Autodesk Inventor part; units mm, degrees
ref_plane "YZ Plane" through (0, 0, 0) normal (1, 0, 0) x (0, 1, 0)
ref_plane "XZ Plane" through (0, 0, 0) normal (0, 1, 0) x (-1, 0, 0)
ref_plane "XY Plane" through (0, 0, 0) normal (0, 0, 1) x (1, 0, 0)
sketch "Sketch1" plane through (0, 0, 0) normal (0, 0, 1) x (1, 0, 0)
  line L0 (210, -0.4421) -> (210, 134.5579)
  line L1 (210, 134.5579) -> (70, 134.5579)
  line L2 (0, 60) -> (0, 0)
  line L3 (70, 60) -> (0, 60)
  line L4 (0, 60) -> (0, 0)
  line L5 (70, 60) -> (70, 134.5579)
  line L6 (0, 0) -> (24.7692, 0)
  line L7 (70, -0.4421) -> (70, 134.5579) construction
  arc A0 (184.7692, 18.0579) -> (147.7692, 18.0579) centre (166.2692, 18.0579) ccw
  line L8 (147.7692, 0) -> (147.7692, 18.0579)
  line L9 (184.7692, -0.4421) -> (184.7692, 18.0579)
  arc A1 (61.7692, 18.5) -> (24.7692, 18.5) centre (43.2692, 18.5) ccw
  line L10 (24.7692, 0) -> (24.7692, 18.5)
  line L11 (61.7692, 0) -> (61.7692, 18.5)
  line L12 (210, 17.0579) -> (205, 17.0579)
  line L13 (205, 17.0579) -> (205, 82.0579)
  line L14 (205, 82.0579) -> (210, 82.0579)
  line L15 (210, 82.0579) -> (210, 17.0579)
  line L16 (184.7692, -0.4421) -> (210, -0.4421)
  line L17 (61.7692, 0) -> (147.7692, 0)
  dimension "d14" = 210
  dimension "d15" = 70
  dimension "d17" = 37
  dimension "d19" = 37
  dimension "d23" = 5
  dimension "d24" = 65
  dimension "d28" = 52.5
  dimension "d48" = 135
  dimension "d51" = 18.5
  dimension "d52" = 18.5
  dimension "d54" = 18.5
  dimension "d55" = 60
  dimension "d60" = 18.5
  dimension "d61" = 123
extrude "Extrusion1" add sketch "Sketch1" along normal blind 5 contours L16 L9 A0 L8 L17 L11 A1 L10 L6 L2 L3 L5 L1 L0 L14 L13 L12
sketch "Sketch2" plane through (0, 0, 5) normal (0, 0, 1) x (1, 0, 0)
  line L0 (205, 17.0579) -> (205, 82.0579)
  line L1 (210, 17.0579) -> (205, 17.0579)
  point P0 (0, 0)
  point P1 (190, 49.5579)
  dimension "d36" = 15
  dimension "d37" = 32.5
hole "Hole1" at (190, 49.5579, 5) direction (0, 0, -1) diameter 3 end through all
sketch "Sketch3" plane through (0, 0, 5) normal (0, 0, 1) x (1, 0, 0)
  line L0 (70, 134.5579) -> (70, 60)
  line L1 (70, 60) -> (0, 60)
  point P0 (0, 0)
  point P1 (75, 90)
  dimension "d45" = 5
  dimension "d46" = 30
hole "Hole2" at (75, 90, 5) direction (0, 0, -1) diameter 3 end through all
properties part number "SIDE_1" material "ABS Plastic"
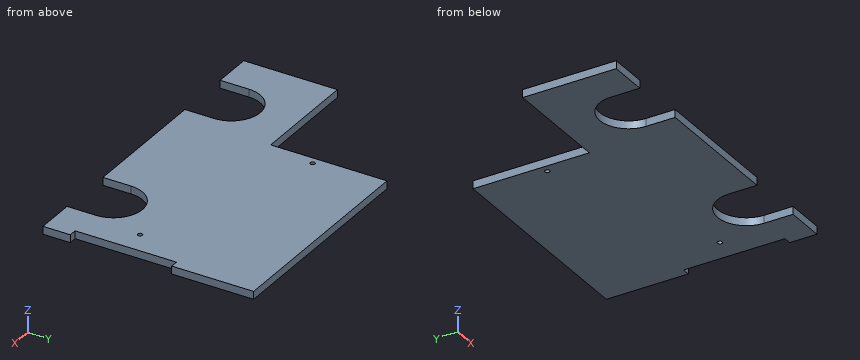
Here's how the part is built. I have some questions about the finished solid (model axes, mm). Round coordinates to 2 decimals unless told otherwise and drop trailing zeros. Order: outer loops, then holes, each group sorted by start corner. A loop starts at its lowest first (then second) coordinate and runs counter-clockwise, first axis right, second up. Notation, with made-up numbers: M 17,-29.5 L 26,-29.5 A20 ccw 26,-19.5 Z; hole C 8.25,36 d9. An arc over 180 degrees is marked long. Answer in a Markdown table with one row per item.
Item 1: If I drill on L1, parallel to Y at x = 75, z = 2.3; L2, parallel to X at y = 27, z = 1.55; L3, parallel to Y at x = 190, z = 1.1, over which ranges is the centre line in solid material (lowest first)? Write a range as from..to.
A:
| item | result |
|---|---|
| L1 | y = 0..88.5, 91.5..134.56 |
| L2 | x = 0..26.84, 59.7..150.07, 182.46..205 |
| L3 | y = -0.44..48.06, 51.06..134.56 |
Item 2: I'm going to push flat-ended pins straight in: pin 1 (2.5 mm diameter, centred on x = 24.5, z = 1.5, fed in from +Y); pin 2 (1.5 mm diameter, centred on y = 82, z = 2, fed in from -X). Where does each tip first touch, or does it pass through?
A:
| item | result |
|---|---|
| pin 1 | stops at y = 60 |
| pin 2 | stops at x = 70 |
Item 3: Imagine slicing it at C-C, the plane y = 109. Write out the boundary of the cut face in (x, z), and give its area (3 significant figures).
A:
| item | result |
|---|---|
| outline | M 70,0 L 210,0 L 210,5 L 70,5 Z |
| area | 700 mm2 |
Item 4: Imagine slicing it at A-A, the plane z = 2.75. Write out the boundary of the cut face in (x, y).
A:
| item | result |
|---|---|
| outline | M 0,0 L 24.77,0 L 24.77,18.5 A18.5 cw 61.77,18.5 L 61.77,0 L 147.77,0 L 147.77,18.06 A18.5 cw 184.77,18.06 L 184.77,-0.44 L 210,-0.44 L 210,17.06 L 205,17.06 L 205,82.06 L 210,82.06 L 210,134.56 L 70,134.56 L 70,60 L 0,60 Z; hole C 75,90 d3; hole C 190,49.56 d3 |
Item 5: Imagine slicing it at B-B, the plane y = 22. Write out the boundary of the cut face in (x, z), and give its area (3 significant figures).
A:
| item | result |
|---|---|
| outline | M 0,0 L 25.1,0 L 25.1,5 L 0,5 Z; M 61.44,0 L 148.19,0 L 148.19,5 L 61.44,5 Z; M 184.34,0 L 205,0 L 205,5 L 184.34,5 Z |
| area | 663 mm2 |
